Here's how the part is built. I have some questions about the finished solid (model axes, mm). A direction names the side the tool comes from. Coordinates: 2 decimals unless noted, no trailing zeros. Loops run counter-clockwise (first coordinate to the right, second up) from the corner with the lowest first, then second, coordinate; pieces in that order, holes last. Notation, with made-up numbers: (-21.75, 65) -> (17.25, 65) arc R8 cw to (17.25, 79) -> close; hole circle Ø7 at (1.5, 33.25). An arc over 180 degrees is marked (long way). Answer as a JSON object with one key per item and string values. Group by question number.
Q1. I want a section at D-D on x = 66. Write out the boundary of the cut face in (y, z).
Q2. Thinking about a two-plate mould opening in X: for faces 6 (the flat face through (41, 28.8, 1)), 7 (the flat face through (80, 17, 4)), 8 (the flat face through (30.56, 12.46, 2.22)), 9 (the flat face through (46.595, 7.52, 2.218)), which applies, released by +X, released by -X, zero draft, split by the parting line, or undercut?
Q3. I'm going to push flat-ended pins straight in: pin 1 (3.5 mm diameter, centred on x = 32, y = 10, fed in from -Z); pin 2 (3 mm diameter, centred on x = 60, y = 25, fed in from +Z); pin 3 (0.5 mm diameter, centred on x = 29, z = 2, fed in from +Y); pin 4 (1.4 mm diameter, centred on x = 47, y = 33.5, fed in from -Z). Where does each tip first touch, or does it pass through?
Q4. On a 3-axis mill with a long thin cutter (end or side, diameter ignored), from which of +Z, -Z, +X, -X, +Y, -Y can I reach the whole of each face in a straight line? I mean faces 1 (the flat face through (33.44, 7.54, 2.22)), 2 (the flat face through (40, 33.2, 3)), 3 (the cylindrical face through (12.45, 11.93, 3.94)), 4 (the flat face through (39, 15, 0)), 5 (the flat face through (41, 33, 2.5)). Say none if no direction works.
Q5. I want a section at C-C on x = 40. Write out the boundary of the cut face in (y, z), then the cut area to 3 significant figures.
Q6. I want a section at B-B on y = 25. Write out the boundary of the cut face in (x, z).
Q7. I want a section at A-A on z = 6.5. Count the separate pieces of the cut face and the enclosed holes in it, then the cut area to 3 significant figures.
Q8. I need wall thicknesses on line 1 (Y direction, x = 48, z = 6.5); line 2 (Y direction, x = 20, z = 6); line 3 (Z direction, x = 28.5, y = 29). Which ranges of each line are inside material? Lowest first, please.
```python
from build123d import *

# Parameters (mm, degrees)
SKETCH_2_W           = 80
SKETCH_2_H           = 34
SKETCH_2_R           = 6
SKETCH_2_R_2         = 4.05
EXTRUDE_1_DEPTH      = 8
CUT_EXTRUDE_2_DEPTH  = 88.292611371
SKETCH_5_R           = 1.55
CUT_EXTRUDE_3_DEPTH  = 88.292611371
CUT_EXTRUDE_5_DEPTH  = 4.5
SKETCH_11_R          = 1.55
CUT_EXTRUDE_7_DEPTH  = 88.292611371
CUT_EXTRUDE_11_DEPTH = 2
SKETCH_22_R          = 1.55
CUT_EXTRUDE_13_DEPTH = 88.292611371


with BuildPart() as part:
    # 草图2 → 凸台-拉伸1 (new body)
    with BuildSketch(Plane.XY):
        with Locations((40, 17)):
            Rectangle(SKETCH_2_W, SKETCH_2_H)
        with Locations((7, 8)):
            Circle(SKETCH_2_R, mode=Mode.SUBTRACT)
        with Locations((40, 10)):
            Circle(SKETCH_2_R_2, mode=Mode.SUBTRACT)
        with Locations((73, 8)):
            Circle(SKETCH_2_R, mode=Mode.SUBTRACT)
    extrude(amount=EXTRUDE_1_DEPTH)

    # 草图4 → 切除-拉伸2 (cut, through all)
    with BuildSketch(Plane(origin=(80, 0, 0), x_dir=(0, 0, -1), z_dir=(1, 0, 0))):
        Polygon((-1.5, 32.2), (-2.5, 32.2), (-2.5, 34), (0, 34), (0, 28.8), (-1.5, 28.8), align=None)
    extrude(amount=-CUT_EXTRUDE_2_DEPTH, mode=Mode.SUBTRACT)

    # 草图5 → 切除-拉伸3 (cut, through all)
    with BuildSketch(Plane.XY.offset(8)):
        with Locations((48, 10)):
            Circle(SKETCH_5_R)
        with Locations((32, 10)):
            Circle(SKETCH_5_R)
    extrude(amount=-CUT_EXTRUDE_3_DEPTH, mode=Mode.SUBTRACT)

    # 草图8 → 切除-拉伸5 (cut)
    with BuildSketch(Plane(origin=(0, 0, 0), x_dir=(-1, 0, 0), z_dir=(0, 0, -1))):
        Polygon((-45.15, 8.354551733), (-45.15, 11.645448267), (-48, 13.290896534), (-50.85, 11.645448267), (-50.85, 8.354551733), (-48, 6.709103466), align=None)
        Polygon((-34.85, 8.354551733), (-32, 6.709103466), (-29.15, 8.354551733), (-29.15, 11.645448267), (-32, 13.290896534), (-34.85, 11.645448267), align=None)
    extrude(amount=-CUT_EXTRUDE_5_DEPTH, mode=Mode.SUBTRACT)

    # 草图11 → 切除-拉伸7 (cut, through all)
    with BuildSketch(Plane(origin=(0, 0, 0), x_dir=(-1, 0, 0), z_dir=(0, 0, -1))):
        with Locations((-60, 25)):
            Circle(SKETCH_11_R)
        with Locations((-20, 25)):
            Circle(SKETCH_11_R)
    extrude(amount=-CUT_EXTRUDE_7_DEPTH, mode=Mode.SUBTRACT)

    # 草图19 → 切除-拉伸11 (cut)
    with BuildSketch(Plane(origin=(0, 0, 2.5), x_dir=(-1, 0, 0), z_dir=(0, 0, -1))):
        with BuildLine():
            Line((-25, 34), (-55.247938178, 34))
            Line((-55.247938178, 34), (-55.247938178, 33.2))
            ThreePointArc((-55.247938178, 33.2), (-54.747938178, 32.7), (-54.247938178, 33.2))
            Line((-54.247938178, 33.2), (-26, 33.2))
            ThreePointArc((-26, 33.2), (-25.5, 32.7), (-25, 33.2))
            Line((-25, 33.2), (-25, 34))
        make_face()
    extrude(amount=-CUT_EXTRUDE_11_DEPTH, mode=Mode.SUBTRACT)

    # 草图22 → 切除-拉伸13 (cut, through all)
    with BuildSketch(Plane(origin=(0, 0, 0), x_dir=(-1, 0, 0), z_dir=(0, 0, -1))):
        with Locations((-66, 12)):
            Circle(SKETCH_22_R)
        with Locations(Location((-14, 12, 0), (0, 0, 180))):
            Circle(SKETCH_22_R)
    extrude(amount=-CUT_EXTRUDE_13_DEPTH, mode=Mode.SUBTRACT)


solid = part.part
```
Result set:
{
 "1": {"outline": "(0, 0) -> (10.45, 0) -> (10.45, 8) -> (0, 8) -> close; (13.55, 0) -> (28.8, 0) -> (28.8, 1.5) -> (32.2, 1.5) -> (32.2, 2.5) -> (34, 2.5) -> (34, 8) -> (13.55, 8) -> close"},
 "2": {"face 6": "zero draft", "face 7": "released by +X", "face 8": "undercut", "face 9": "undercut"},
 "3": {"pin 1": "stops at z = 4.5", "pin 2": "passes through", "pin 3": "stops at y = 32.2", "pin 4": "stops at z = 2.5"},
 "4": {"face 1": "-Z", "face 2": "-Z, +Y", "face 3": "+Z, -Z", "face 4": "-Z, +X, -X, +Y, -Y", "face 5": "-Z, +X, -X, +Y"},
 "5": {"outline": "(0, 0) -> (5.95, 0) -> (5.95, 8) -> (0, 8) -> close; (14.05, 0) -> (28.8, 0) -> (28.8, 1.5) -> (32.2, 1.5) -> (32.2, 2.5) -> (33.2, 2.5) -> (33.2, 4.5) -> (34, 4.5) -> (34, 8) -> (14.05, 8) -> close", "area": "196 mm²"},
 "6": {"outline": "(0, 0) -> (18.45, 0) -> (18.45, 8) -> (0, 8) -> close; (21.55, 0) -> (58.45, 0) -> (58.45, 8) -> (21.55, 8) -> close; (61.55, 0) -> (80, 0) -> (80, 8) -> (61.55, 8) -> close"},
 "7": {"separate pieces": "1", "enclosed holes": "9", "area": "2,400 mm²"},
 "8": {"line 1": "y = 0 to 8.45, 11.55 to 34", "line 2": "y = 0 to 23.45, 26.55 to 34", "line 3": "z = 1.5 to 8"}
}
